Can you work these out from the model? Positions are in its coordinate system, mm. A direction names the side the tool comes from. Give positions to 0.01 mm unless a question says otherwise; leave off trailing zeros. Order: outer loops, then holes, each group sorted by start corner. A loop starts at its lowest first (then second) coordinate and runs counter-clockwise, first axis right, second up.
Item 1: If I drill on line 1 along Y through (x, z) = (-83.5, -12); line 2 along X through (y, z) = (55, 21); line 3 along X through (y, z) = (-12, -13.5), over which ranges is the centre line in solid material (lowest first)?
Item 2: If we mould it in two halves opening along Y, with no side actions, what happens to faces 1 (the flat face through (-6, -62, 8.15)), 2 (the cylindrical face through (-0.9, 61.97, 18.22)), 3 (the flat face through (90, -31.75, -13))? For each: +Y half, -Y half, draft (parallel to the pull), parting line (faces both ways), or undercut.
Item 3: I want a section at C-C, the plane z = 1. Count the separate pieces of the cut face and the enclosed holes in it, then the cut area to 3 significant figures.
Item 4: I want a section at B-B, the plane x = -29. Write out the boundary of the cut face in (y, z) (3 decimals).
Item 5: Which directions (+Z, -Z, +X, -X, +Y, -Y) give clear straight access to the entire face, cutting with the end or side of a thin tool? Please do faces 4 (the flat face through (-100, -58, 27.051)), 5 (the cylindrical face through (70.08, -31, -0.18)), 6 (the cylindrical face through (0.9, -61.97, -18.51)), 7 (the cylindrical face through (0.919, 63.493, -18.506)), 8 (the flat face through (91, 31.75, -13)).
Item 6: I'm going to push flat-ended pins straight in: pin 1 Ø1.2 at (y, z) = (31, 27.5) entering from +X; pin 2 Ø3 at (x, z) = (53.5, 7) entering from +Y; pin 3 Ø5 at (y, z) = (48.5, -13.5) entering from +X (3 decimals). Where does each tip first touch, or does it pass through?
Item 7: I want a section at A-A, the plane y = -52. Write out the boundary of the cut face in (x, z) (3 decimals).
Item 8: I want a section at D-D, the plane y = -12. Write out the boundary of the cut face in (x, z) (3 decimals), then the cut area to 3 significant figures.
```python
from build123d import *

# Parameters (mm, degrees)
BASE_FLANGE1_START            = -28.575
BASE_FLANGE1_DEPTH            = 57.15
EDGE_FLANGE2_STRIP_W          = 9.144
EDGE_FLANGE2_STRIP_H          = 1.524
EDGE_FLANGE2_STRIP_CUT_DEPTH  = 44.45
EDGE_FLANGE2_RELIEF_W         = 9.906
EDGE_FLANGE2_RELIEF_H         = 0.762
EDGE_FLANGE2_RELIEF_CUT_DEPTH = 1.524
EDGE_FLANGE2_DEPTH            = 44.45
EDGE_FLANGE2_PROFILE_W        = 44.45
EDGE_FLANGE2_PROFILE_H        = 49.276
EDGE_FLANGE2_PROFILE_R        = 9.525
EDGE_FLANGE2_FLAT_DEPTH       = 1.524
HEM1_START                    = -28.575
HEM1_DEPTH                    = 57.15
HEM1_2_DEPTH                  = 57.15
SKETCH22_R                    = 12.7
CUT_EXTRUDE1_DEPTH            = 174.234005394
CUT_EXTRUDE2_DEPTH            = 174.234005394
CUT_EXTRUDE2_DEPTH_BACK       = 174.234005394


with BuildPart() as part:
    # Base-Flange1: read off the stored shape, not the designer's step
    # Base-Flange1 outline → Base-Flange1 (new body)
    with BuildSketch(Plane.XY.offset(BASE_FLANGE1_START)):
        with BuildLine():
            Line((55.865566318, 30.226), (127, 30.226))
            Line((127, 30.226), (127, 31.75))
            Line((127, 31.75), (55.865566318, 31.75))
            ThreePointArc((55.865566318, 31.75), (55.11254895, 31.949031757), (54.556217107, 32.494140625))
            ThreePointArc((54.556217107, 32.494140625), (0, 63.5), (-54.556217107, 32.494140625))
            ThreePointArc((-54.556217107, 32.494140625), (-55.11254895, 31.949031757), (-55.865566318, 31.75))
            Line((-55.865566318, 31.75), (-123.952, 31.75))
            ThreePointArc((-123.952, 31.75), (-126.107261469, 30.857261469), (-127, 28.702))
            Line((-127, 28.702), (-127, -28.702))
            ThreePointArc((-127, -28.702), (-126.107261469, -30.857261469), (-123.952, -31.75))
            Line((-123.952, -31.75), (-55.865566318, -31.75))
            ThreePointArc((-55.865566318, -31.75), (-55.11254895, -31.949031757), (-54.556217107, -32.494140625))
            ThreePointArc((-54.556217107, -32.494140625), (0, -63.5), (54.556217107, -32.494140625))
            ThreePointArc((54.556217107, -32.494140625), (55.11254895, -31.949031757), (55.865566318, -31.75))
            Line((55.865566318, -31.75), (127, -31.75))
            Line((127, -31.75), (127, -30.226))
            Line((127, -30.226), (55.865566318, -30.226))
            ThreePointArc((55.865566318, -30.226), (54.359531582, -30.624063515), (53.246867897, -31.71428125))
            ThreePointArc((53.246867897, -31.71428125), (0, -61.976), (-53.246867897, -31.71428125))
            ThreePointArc((-53.246867897, -31.71428125), (-54.359531582, -30.624063515), (-55.865566318, -30.226))
            Line((-55.865566318, -30.226), (-123.952, -30.226))
            ThreePointArc((-123.952, -30.226), (-125.029630735, -29.779630735), (-125.476, -28.702))
            Line((-125.476, -28.702), (-125.476, 28.702))
            ThreePointArc((-125.476, 28.702), (-125.029630735, 29.779630735), (-123.952, 30.226))
            Line((-123.952, 30.226), (-55.865566318, 30.226))
            ThreePointArc((-55.865566318, 30.226), (-54.359531582, 30.624063515), (-53.246867897, 31.71428125))
            ThreePointArc((-53.246867897, 31.71428125), (0, 61.976), (53.246867897, 31.71428125))
            ThreePointArc((53.246867897, 31.71428125), (54.359531582, 30.624063515), (55.865566318, 30.226))
        make_face()
    extrude(amount=BASE_FLANGE1_DEPTH)

    # Edge-Flange2: sheet metal written as solids
    # Edge-Flange2 strip (on a plane across the edge) → Edge-Flange2 strip cut (cut)
    with BuildSketch(Plane(origin=(-112.365340231, 31.75, 28.575), x_dir=(0, 0, -1), z_dir=(1, 0, 0))):
        with Locations((-1.524, -0.762)):
            Rectangle(EDGE_FLANGE2_STRIP_W, EDGE_FLANGE2_STRIP_H)
    edge_flange2_strip_cut = extrude(amount=EDGE_FLANGE2_STRIP_CUT_DEPTH, mode=Mode.SUBTRACT)

    # Edge-Flange2 relief (on the sheet) → Edge-Flange2 relief cut (cut)
    with BuildSketch(Plane(origin=(-112.365340231, 31.75, 25.527), x_dir=(0, 0, -1), z_dir=(0, 1, 0))):
        with Locations((-4.191, 0.381)):
            Rectangle(EDGE_FLANGE2_RELIEF_W, EDGE_FLANGE2_RELIEF_H)
        with Locations((-4.191, -44.831)):
            Rectangle(EDGE_FLANGE2_RELIEF_W, EDGE_FLANGE2_RELIEF_H)
    edge_flange2_relief_cut = extrude(amount=-EDGE_FLANGE2_RELIEF_CUT_DEPTH, mode=Mode.SUBTRACT)

    # Edge-Flange2 bend section (on a plane across the edge) → Edge-Flange2 (add)
    with BuildSketch(Plane(origin=(-112.365340231, 31.75, 28.575), x_dir=(0, 0, -1), z_dir=(1, 0, 0))):
        with BuildLine():
            Line((0, 1.524), (1.524, 1.524))
            ThreePointArc((1.524, 1.524), (1.970369265, 0.446369265), (3.048, 0))
            Line((3.048, 0), (3.048, -1.524))
            ThreePointArc((3.048, -1.524), (0.892738531, -0.631261469), (0, 1.524))
        make_face()
    edge_flange2 = extrude(amount=EDGE_FLANGE2_DEPTH)

    # Edge-Flange2 profile (on flange) → Edge-Flange2 flat (add)
    with BuildSketch(Plane(origin=(0, 31.75, 28.575), x_dir=(1, 0, 0), z_dir=(0, 0, 1))):
        with Locations((-90.140340231, 26.162)):
            Rectangle(EDGE_FLANGE2_PROFILE_W, EDGE_FLANGE2_PROFILE_H)
        with Locations((-90.140340231, 25.4)):
            Circle(EDGE_FLANGE2_PROFILE_R, mode=Mode.SUBTRACT)
    edge_flange2_flat = extrude(amount=-EDGE_FLANGE2_FLAT_DEPTH)

    # Mirror1: Edge-Flange2 strip cut, Edge-Flange2 relief cut, Edge-Flange2, Edge-Flange2 flat across plane
    add(edge_flange2_strip_cut.mirror(Plane.ZX), mode=Mode.SUBTRACT)
    add(edge_flange2_relief_cut.mirror(Plane.ZX), mode=Mode.SUBTRACT)
    add(edge_flange2.mirror(Plane.ZX))
    add(edge_flange2_flat.mirror(Plane.ZX))

    # Hem1: read off the stored shape, not the designer's step
    # Hem1 outline → Hem1 (cut)
    with BuildSketch(Plane.XY.offset(HEM1_START)):
        with BuildLine():
            ThreePointArc((125.095, 31.75), (126.299827788, 31.320606655), (126.961511183, 30.226))
            Line((126.961511183, 30.226), (127, 30.226))
            Line((127, 30.226), (127, 31.75))
            Line((127, 31.75), (125.095, 31.75))
        make_face()
        with BuildLine():
            Line((127, -30.226), (126.961511183, -30.226))
            ThreePointArc((126.961511183, -30.226), (126.299827788, -31.320606655), (125.095, -31.75))
            Line((125.095, -31.75), (127, -31.75))
            Line((127, -31.75), (127, -30.226))
        make_face()
    extrude(amount=HEM1_DEPTH, mode=Mode.SUBTRACT)

    # Hem1 2 outline → Hem1 2 (add)
    with BuildSketch(Plane.XY.offset(HEM1_START)):
        with BuildLine():
            Line((123.122180151, 30.157595971), (122.600941452, 28.725504417))
            Line((122.600941452, 28.725504417), (124.443451627, 28.054885557))
            ThreePointArc((124.443451627, 28.054885557), (126.338972724, 28.402239846), (126.961511183, 30.226))
            Line((126.961511183, 30.226), (125.095, 30.226))
            ThreePointArc((125.095, 30.226), (125.470211754, 29.778840044), (124.964690325, 29.486977111))
            Line((124.964690325, 29.486977111), (123.122180151, 30.157595971))
        make_face()
        with BuildLine():
            Line((122.600941452, -28.725504417), (123.122180151, -30.157595971))
            Line((123.122180151, -30.157595971), (124.964690325, -29.486977111))
            ThreePointArc((124.964690325, -29.486977111), (125.470211754, -29.778840044), (125.095, -30.226))
            Line((125.095, -30.226), (126.961511183, -30.226))
            ThreePointArc((126.961511183, -30.226), (126.338972724, -28.402239846), (124.443451627, -28.054885557))
            Line((124.443451627, -28.054885557), (122.600941452, -28.725504417))
        make_face()
    extrude(amount=HEM1_2_DEPTH)

    # Sketch22 → Cut-Extrude1 (cut, through all)
    with BuildSketch(Plane(origin=(0, 31.75, 0), x_dir=(1, 0, 0), z_dir=(0, 1, 0))):
        with Locations(Location((90.480283159, 0, 0), (0, 0, 90))):
            Circle(SKETCH22_R)
    extrude(amount=-CUT_EXTRUDE1_DEPTH, mode=Mode.SUBTRACT)

    # Sketch23 → Cut-Extrude2 (cut, two sides: drawn at the far end of the back side and taken through both)
    with BuildSketch(Plane(origin=(0, 31.75, 0), x_dir=(1, 0, 0), z_dir=(0, 1, 0)).offset(-CUT_EXTRUDE2_DEPTH_BACK)):
        with BuildLine():
            Line((-65.067682155, 8.15016142), (61.932317845, 8.15016142))
            ThreePointArc((61.932317845, 8.15016142), (70.082479265, 0), (61.932317845, -8.15016142))
            Line((61.932317845, -8.15016142), (-65.067682155, -8.15016142))
            ThreePointArc((-65.067682155, -8.15016142), (-73.217843575, 0), (-65.067682155, 8.15016142))
        make_face()
    extrude(amount=CUT_EXTRUDE2_DEPTH + CUT_EXTRUDE2_DEPTH_BACK, mode=Mode.SUBTRACT)


solid = part.part
```
Results list:
1. line 1: y = -31.75 to -30.23, 30.23 to 31.75
1. line 2: x = -31.74 to -28.57, 28.57 to 31.74
1. line 3: x = -127 to -125.48
2. face 1: draft
2. face 2: undercut
2. face 3: -Y half
3. separate pieces: 5
3. enclosed holes: 0
3. area: 362 mm2
4. outline: (-56.491, -28.575) - (-54.772, -28.575) - (-54.772, -8.15) - (-56.491, -8.15) - close; (-56.491, 8.15) - (-54.772, 8.15) - (-54.772, 28.575) - (-56.491, 28.575) - close; (54.772, -28.575) - (56.491, -28.575) - (56.491, -8.15) - (54.772, -8.15) - close; (54.772, 8.15) - (56.491, 8.15) - (56.491, 28.575) - (54.772, 28.575) - close
5. face 4: -Z, -X, -Y
5. face 5: +Y, -Y
5. face 6: +Z, -Z
5. face 7: +Z, -Z, +Y
5. face 8: +Z, -Z, +X, +Y
6. pin 1: stops at x = 126.92
6. pin 2: stops at y = 35.67
6. pin 3: stops at x = 43.775
7. outline: (-112.365, 27.051) - (-98.153, 27.051) - (-98.153, 28.575) - (-112.365, 28.575) - close; (-82.128, 27.051) - (-67.915, 27.051) - (-67.915, 28.575) - (-82.128, 28.575) - close; (-36.445, -28.575) - (-33.72, -28.575) - (-33.72, -8.15) - (-36.445, -8.15) - close; (-36.445, 8.15) - (-33.72, 8.15) - (-33.72, 28.575) - (-36.445, 28.575) - close; (33.72, -28.575) - (36.445, -28.575) - (36.445, -8.15) - (33.72, -8.15) - close; (33.72, 8.15) - (36.445, 8.15) - (36.445, 28.575) - (33.72, 28.575) - close
8. outline: (-127, -28.575) - (-125.476, -28.575) - (-125.476, 28.575) - (-127, 28.575) - close
8. area: 87.1 mm2
